from build123d import *

# Parameters (mm, degrees)
SKETCH_W      = 21.8
SKETCH_H      = 7
PAD_DEPTH     = 10.5
THICKNESS_T   = 2
SKETCH001_W   = 25.8
SKETCH001_H   = 11
SKETCH001_W_2 = 21.8
SKETCH001_H_2 = 8.3
PAD001_DEPTH  = 6
SKETCH002_W   = 3.3
SKETCH002_H   = 1.35
POCKET_DEPTH  = 6
CHAMFER_SIZE  = 1


with BuildPart() as part:
    # Sketch → Pad (new body)
    with BuildSketch(Plane.XY):
        Rectangle(SKETCH_W, SKETCH_H)
    extrude(amount=PAD_DEPTH)

    # Thickness
    thickness_openings = [part.faces().sort_by_distance(p)[0] for p in [
        (0, 0, 10.5),
    ]]
    offset(amount=THICKNESS_T, openings=thickness_openings, kind=Kind.INTERSECTION)

    # Sketch001 (on Face6 of Thickness) → Pad001 (join)
    with BuildSketch(Plane.XY.offset(10.5)):
        Rectangle(SKETCH001_W, SKETCH001_H)
        Rectangle(SKETCH001_W_2, SKETCH001_H_2, mode=Mode.SUBTRACT)
    extrude(amount=PAD001_DEPTH)

    # Sketch002 (on Face8 of Pad001) → Pocket (cut)
    with BuildSketch(Plane.XY.offset(16.5)):
        with Locations((-4.25, 4.825)):
            Rectangle(SKETCH002_W, SKETCH002_H)
    extrude(amount=-POCKET_DEPTH, mode=Mode.SUBTRACT)

    # Chamfer
    chamfer_edges = [part.edges().sort_by_distance(p)[0] for p in [
        (-12.9, -5.5, 7.25),
        (12.9, -5.5, 7.25),
        (-12.9, 5.5, 7.25),
        (12.9, 5.5, 7.25),
        (-12.9, 0, -2),
        (0, -5.5, -2),
        (0, 5.5, -2),
        (12.9, 0, -2),
    ]]
    chamfer(chamfer_edges, length=CHAMFER_SIZE)


solid = part.part
Build history of the part. All positions in model axes, mm. A direction names the side the tool comes from. Give positions to 0.01 mm unless a question says otherwise; leave off trailing zeros. Order: outer loops, then holes, each group sorted by start corner. A loop starts at its lowest first (then second) coordinate and runs counter-clockwise, first axis right, second up. Notation, with made-up numbers: M 58.25,55 L 102.25,55 A30 ccw 102.25,79 Z; hole C 7.25,-3.5 d9. An arc over 180 degrees is marked long. Put each result on its own line as item: value.
Item 1: Cut at D-D on y = -1.25. Write the cut outline in (x, z).
Results are:
outline: M -12.9,-1 L -11.9,-2 L 11.9,-2 L 12.9,-1 L 12.9,16.5 L 10.9,16.5 L 10.9,0 L -10.9,0 L -10.9,16.5 L -12.9,16.5 Z
Item 2: Cut at C-C on z = 11.75. Write the cut outline in (x, y).
Results are:
outline: M -12.9,-4.5 L -11.9,-5.5 L 11.9,-5.5 L 12.9,-4.5 L 12.9,4.5 L 11.9,5.5 L -2.6,5.5 L -2.6,4.15 L 10.9,4.15 L 10.9,-4.15 L -10.9,-4.15 L -10.9,4.15 L -5.9,4.15 L -5.9,5.5 L -11.9,5.5 L -12.9,4.5 Z
Item 3: Wall check: probe 1 along Y at (x, z) = (-0.5, 10); probe 2 along X at (y, z) = (1.75, 11.25); probe 3 along Y at (x, z) = (1.75, 14.25). Give the ranges that are in metal, low to high.
Results are:
probe 1: -5.5 to -3.5, 3.5 to 5.5
probe 2: -12.9 to -10.9, 10.9 to 12.9
probe 3: -5.5 to -4.15, 4.15 to 5.5
Item 4: Pull direction Y, two halves, no side cores. Call faces 1 (the face through (0, -4.15, 13)), 2 (the face through (-0.2, 5, -1.5)), 3 (the face through (-8, 4.15, 13)), 4 (the face through (0, -5, 16.5)): +Y half, -Y half, draft (parallel to the pull), parting line (faces both ways), or undercut.
Results are:
face 1: undercut
face 2: +Y half
face 3: undercut
face 4: draft
Item 5: Which spindle directions (+Z, -Z, +X, -X, +Y, -Y) get a long thin tool onto all of the face, cutting with end or side? Do faces 5 (the face through (4, 4.15, 13)), 6 (the face through (-2.6, 5, 14)), 7 (the face through (12.2, -4.8, -1.4)). Say none if no direction does.
Results are:
face 5: +Z
face 6: +Z, +Y
face 7: -Z, +X, -Y
Item 6: Drop a flat-ended pin along its axis: pin 1 Ø3.5 at (x, y) = (-3.5, 0.5) entering from +Z. Give the stop position or say it passes through.
Results are:
pin 1: z = 0
Item 7: Cut at B-B on x = 2. Write the cut outline in (y, z).
Results are:
outline: M -5.5,-1 L -4.5,-2 L 4.5,-2 L 5.5,-1 L 5.5,16.5 L 4.15,16.5 L 4.15,10.5 L 3.5,10.5 L 3.5,0 L -3.5,0 L -3.5,10.5 L -4.15,10.5 L -4.15,16.5 L -5.5,16.5 Z
Item 8: Cut at A-A on z = 1.75. Write the cut outline in (x, y), then the cut area to 3 significant figures.
Results are:
outline: M -12.9,-4.5 L -11.9,-5.5 L 11.9,-5.5 L 12.9,-4.5 L 12.9,4.5 L 11.9,5.5 L -11.9,5.5 L -12.9,4.5 Z; hole M -10.9,-3.5 L 10.9,-3.5 L 10.9,3.5 L -10.9,3.5 Z
area: 129 mm2
